from build123d import *

# Parameters (mm, degrees)
ESQUISSE1_R        = 9.4
BOSS_EXTRU_1_DEPTH = 5


with BuildPart() as part:
    # Esquisse1 → Boss.-Extru.1 (new body)
    with BuildSketch(Plane.XY):
        Polygon((90, 45), (34.5, 45), (-34.5, 45), (-90, 45), (-90, 37.5), (-87, 37.5), (-87, 24), (-85, 24), (-85, 25.1), (-82.7, 25.1), (-82.7, 24), (-75, 24), (-75, 21), (-82.7, 21), (-82.7, 19.9), (-85, 19.9), (-85, 21), (-87, 21), (-87, 7.5), (-90, 7.5), (-90, 0), (90, 0), (90, 7.5), (87, 7.5), (87, 21), (85, 21), (85, 19.9), (82.7, 19.9), (82.7, 21), (75, 21), (75, 24), (82.7, 24), (82.7, 25.1), (85, 25.1), (85, 24), (87, 24), (87, 37.5), (90, 37.5), align=None)
        with Locations((0, 21)):
            Circle(ESQUISSE1_R, mode=Mode.SUBTRACT)
    extrude(amount=BOSS_EXTRU_1_DEPTH)


solid = part.part
Geometry: final body of the model. Coordinates: model frame, mm. A direction names the side the tool comes from. Round coordinates to 2 decimals unless told otherwise and drop trailing zeros. Write each loop counter-clockwise with the first axis right and the second up, starting at its lowest first coordinate (ties: lowest second). Pieces come first, ordered by that corner, then holes. Notation, with made-up numbers: M 53,3.5 L 88,3.5 A25 cw 88,38.5 Z; hole C 70.25,39 d4. An arc over 180 degrees is marked long. Write item = value, one per line.
Item 1: Section query B-B on y = 35. Return loops of the section in (x, z).
Findings:
outline = M -87,0 L 87,0 L 87,5 L -87,5 Z
Item 2: Pull-direction query (Y, two-part tool) for faces 1 (the face through (90, 41, 2)), 2 (the face through (88, 37.5, 2)); classes: pulls with the +Y half, pulls with the -Y half, needs draft (parallel to the pull), parting line crosses it, or undercut.
Findings:
face_1 = needs draft
face_2 = undercut
Item 3: Access query for faces 3 (the face through (-88, 7.5, 2)), 4 (the face through (-1, 33, 0)), 5 (the face through (87, 31, 2)). Directions: +Z, -Z, +X, -X, +Y, -Y. A direction counts if a zero-diameter tool reaches every point of the face in a straight line with its end or side. Return the directions, or none.
Findings:
face_3 = +Z, -Z, -X
face_4 = -Z, +X, -X, +Y, -Y
face_5 = +Z, -Z, +X
Item 4: Pin query (flat end, axial travel): P1, Ø0.9, axis at y = 24.5, z = 3, coming from the -X side; P2, Ø1.8, axis at x = -83.5, z = 2.5, coming from the -Y side; P3, Ø1.5, axis at y = 22, z = 1.5, coming from the +X side; P4, Ø2, axis at y = 10, z = 2, coming from the +X side. Return the tip coordinate at first contact, or that it passes through.
Findings:
P1 = -87
P2 = 0
P3 = 75
P4 = 87
Item 5: Section query A-A on x = 0. Return loops of the section in (y, z).
Findings:
outline = M 0,0 L 11.6,0 L 11.6,5 L 0,5 Z; M 30.4,0 L 45,0 L 45,5 L 30.4,5 Z
Item 6: Material intervals for line 1 along Y through (x, z) = (-82, 0.4); line 2 along Y through (x, z) = (0, 3.4); line 3 along X through (y, z) = (30.5, 3.4), sorted ascending. Write a range as [from, to].
Findings:
line_1 = [0, 21], [24, 45]
line_2 = [0, 11.6], [30.4, 45]
line_3 = [-87, 87]
